```python
from build123d import *

# Parameters (mm, degrees)
CUT_EXTRUDE_1_DEPTH      = 14.97283078
FILLET_1_R               = 1
CUT_EXTRUDE_2_REACH      = 17.831
CUT_EXTRUDE_2_END_RADIUS = 3.4
SKETCH_3_R               = 0.75
SKETCH_4_R               = 2
CUT_EXTRUDE_3_DEPTH      = 2
SKETCH_5_OUTSIDE_W       = 15.602
SKETCH_5_OUTSIDE_H       = 18.902
SKETCH_5_OUTSIDE_R       = 4.7
CUT_EXTRUDE_4_DEPTH      = 1.5
CUT_EXTRUDE_START        = -8.2
SKETCH_5_2_OUTSIDE_W     = 15.602
SKETCH_5_2_OUTSIDE_H     = 18.902
SKETCH_5_2_OUTSIDE_R     = 4.7
CUT_EXTRUDE_5_DEPTH      = 2
CHAMFER_1_SIZE           = 0.5


with BuildPart() as part:
    # Эскиз1 → Повернуть1 (revolve)
    with BuildSketch(Plane(origin=(0, 0, 0), x_dir=(0, 0, -1), z_dir=(1, 0, 0)), mode=Mode.PRIVATE) as revolve_1_sk:
        Polygon((-3.4, 0), (-3.4, 6.5), (-0.9, 6.5), (-0.9, 13.85), (-1.75, 13.85), (-1.75, 8.2), (-8, 8.2), (-8, 0), align=None)
    revolve(revolve_1_sk.sketch.rotate(Axis((0, 0, 0), (0, 1, 0)), 180), axis=Axis((0, 0, 0), (0, 1, 0)))

    # Эскиз2 → Вырез-Вытянуть1 (cut, through all)
    with BuildSketch(Plane(origin=(0, 8.2, 0), x_dir=(1, 0, 0), z_dir=(0, 1, 0))):
        with BuildLine():
            ThreePointArc((7.99025974, -7.116582697), (0, 10.7), (-7.99025974, -7.116582697))
            ThreePointArc((-7.99025974, -7.116582697), (-3.75469644, -7.361538877), (-3.50974026, -3.125975577))
            ThreePointArc((-3.50974026, -3.125975577), (0, 4.7), (3.50974026, -3.125975577))
            ThreePointArc((3.50974026, -3.125975577), (3.75469644, -7.361538877), (7.99025974, -7.116582697))
        make_face()
    extrude(amount=-CUT_EXTRUDE_1_DEPTH, mode=Mode.SUBTRACT)

    # Скругление1
    fillet_1_edges = [part.edges().sort_by_distance(p)[0] for p in [
        (-3.555293146, 4.1, 7.166581517),
        (3.555293146, 4.1, 7.166581517),
    ]]
    fillet(fillet_1_edges, radius=FILLET_1_R)

    # Вырез-Вытянуть2: up to this cylinder (the profile starts outside it)
    cut_extrude_2_end = Plane(origin=(0, 4.1, 0), z_dir=(0, -1, 0)) * Cylinder(CUT_EXTRUDE_2_END_RADIUS, 43.462, mode=Mode.PRIVATE)
    # Эскиз3 → Вырез-Вытянуть2 (cut, up to the surface)
    with BuildSketch(Plane(origin=(0, 8.2, 8), x_dir=(1, 0, 0), z_dir=(0, 0, 1)), mode=Mode.PRIVATE) as cut_extrude_2_sk1:
        with Locations((0, -4.1)):
            Circle(SKETCH_3_R)
    cut_extrude_2_tool1 = extrude(cut_extrude_2_sk1.sketch, amount=-CUT_EXTRUDE_2_REACH, mode=Mode.PRIVATE) - cut_extrude_2_end
    add(cut_extrude_2_tool1.solids().sort_by_distance((0, 4.1, 8))[0], mode=Mode.SUBTRACT)

    # Эскиз4 → Вырез-Вытянуть3 (cut)
    with BuildSketch(Plane(origin=(0, 8.2, 8), x_dir=(1, 0, 0), z_dir=(0, 0, 1))):
        with Locations((0, -4.1)):
            Circle(SKETCH_4_R)
    extrude(amount=-CUT_EXTRUDE_3_DEPTH, mode=Mode.SUBTRACT)

    # Эскиз5 outside → Вырез-Вытянуть4 (cut)
    with BuildSketch(Plane(origin=(0, 8.2, 0), x_dir=(1, 0, 0), z_dir=(0, 1, 0))):
        with Locations((0, -1.65)):
            Rectangle(SKETCH_5_OUTSIDE_W, SKETCH_5_OUTSIDE_H)
        with Locations(Location((0, 0, 0), (0, 0, 270))):
            Circle(SKETCH_5_OUTSIDE_R, mode=Mode.SUBTRACT)
    extrude(amount=-CUT_EXTRUDE_4_DEPTH, mode=Mode.SUBTRACT)

    # Эскиз5<2> outside → Вырез-Вытянуть5 (cut)
    with BuildSketch(Plane(origin=(0, 8.2, 0), x_dir=(1, 0, 0), z_dir=(0, 1, 0)).offset(CUT_EXTRUDE_START)):
        with Locations((0, -1.65)):
            Rectangle(SKETCH_5_2_OUTSIDE_W, SKETCH_5_2_OUTSIDE_H)
        with Locations(Location((0, 0, 0), (0, 0, 270))):
            Circle(SKETCH_5_2_OUTSIDE_R, mode=Mode.SUBTRACT)
    extrude(amount=CUT_EXTRUDE_5_DEPTH, mode=Mode.SUBTRACT)

    # Фаска1
    chamfer_1_edges = [part.edges().sort_by_distance(p)[0] for p in [
        (0, 13.85, 1.75),
    ]]
    chamfer(chamfer_1_edges, length=CHAMFER_1_SIZE)


solid = part.part
```
Geometry: final body of the model. Coordinates: model frame, mm. A direction names the side the tool comes from. Round coordinates to 2 decimals unless told otherwise and drop trailing zeros. Order: outer loops, then holes, each group sorted by start corner. A loop starts at its lowest first (then second) coordinate and runs counter-clockwise, first axis right, second up. Notation, with made-up numbers: (11, 38.5) -> (27, 38.5) arc R15 cw to (27, 50.5) -> close; hole circle Ø5 at (-37, -35.5). An arc over 180 degrees is marked (long way). Use one line per item in the form item = value. Start each with the question number.
1. Line query: probe 1 along X at (y, z) = (3.5, 0); probe 2 along X at (y, z) = (10, 0); probe 3 along Z at (x, y) = (0.25, 7). Output: solid intervals per line, ascending.
2. Cut plane B-B (x = 0). Count the separate pieces of the cut face and the enclosed holes in it, then the cut area to 3 significant figures.
3. Reachability of faces 5 (the face through (-2.786, 4.383, 4.659)), 6 (the face through (1.3, 3.3, -3.14)), 7 (the face through (1.847, 3.334, 7.014)) from +Z, -Z, +X, -X, +Y, -Y: full face, straight path, thin tool, end or side. Return the list, or none.
4. Pin query (flat end, axial travel): pin 1 Ø1.5 at (x, z) = (-1.5, 6.5) entering from +Y; pin 2 Ø3 at (y, z) = (6, -2) entering from +X; pin 3 Ø4 at (x, z) = (0.5, 5) entering from -Y; pin 4 Ø1.1 at (x, z) = (0, 0) entering from +Y. Return the tip coordinate at first contact, or that it passes through.
5. Draft query along Z for faces 1 (the face through (1, 6.5, -1)), 2 (the face through (0.67, 10.739, -1.617)), 3 (the face through (0, 8.2, 2)), 4 (the face through (1, 4, 6)). Return one class per face: pulls with the +Z half, pulls with the -Z half, needs draft (parallel to the pull), parting line crosses it, or undercut.
6. Cut plane A-A (z = 0). Return the cut outline in (x, y), then the cut area to 3 significant figures.
Solution:
q1.probe_1 = -4.7 to -3.4, 3.4 to 4.7
q1.probe_2 = -1.75 to -0.9, 0.9 to 1.75
q1.probe_3 = -4.69 to -0.86, 0.86 to 4.69
q2.separate_pieces = 3
q2.enclosed_holes = 0
q2.area = 42.8 mm^2
q3.face_5 = -X, +Y, -Y
q3.face_6 = -Y
q3.face_7 = +Z
q4.pin_1 = 6.7
q4.pin_2 = 4.67
q4.pin_3 = 0
q4.pin_4 = through
q5.face_1 = undercut
q5.face_2 = parting line crosses it
q5.face_3 = needs draft
q5.face_4 = pulls with the +Z half
q6.outline = (-4.7, 0) -> (-3.4, 0) -> (-3.4, 6.5) -> (-0.9, 6.5) -> (-0.9, 13.85) -> (-1.25, 13.85) -> (-1.75, 13.35) -> (-1.75, 8.2) -> (-4.7, 8.2) -> close; (0.9, 6.5) -> (3.4, 6.5) -> (3.4, 0) -> (4.7, 0) -> (4.7, 8.2) -> (1.75, 8.2) -> (1.75, 13.35) -> (1.25, 13.85) -> (0.9, 13.85) -> close
q6.area = 39.2 mm^2
